Model file for the job. Use its own axes, mm. Give positions to 0.01 mm unless a question says otherwise; leave off trailing zeros. Write each loop counter-clockwise with the first axis right and the second up, starting at its lowest first coordinate (ties: lowest second). Pieces come first, ordered by that corner, then holes. Notation, with made-up numbers: (87, 55) - (100, 55) arc R21 cw to (100, 66) - close; hole circle Ø6 at (41.5, 53). An arc over 180 degrees is marked (long way). Use a Markdown table: item, result. Add a question column.
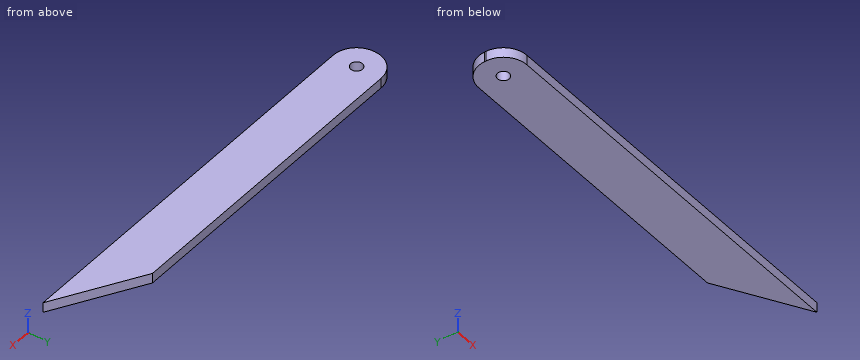
```python
from build123d import *

# Parameters (mm, degrees)
F1_DEPTH = 1.0795
F2_R     = 5.08
F3_R     = 1.27
F4_DEPTH = 25.4


with BuildPart() as f1:
    # F0 (on Top) → F1 (new body, symmetric)
    with BuildSketch(Plane.XY):
        Polygon((0, 10.414), (0, 0), (88.9, 0), (71.12, 10.414), align=None)
    extrude(amount=F1_DEPTH, both=True)

    # F2
    f2_edges = [f1.edges().sort_by_distance(p)[0] for p in [
        (0, 10.414, 0),
        (0, 0, 0),
    ]]
    fillet(f2_edges, radius=F2_R)

    # F3 (on face) → F4 (cut)
    with BuildSketch(Plane.XY.offset(1.0795)):
        with Locations((5.08, 5.08)):
            Circle(F3_R)
    extrude(amount=-F4_DEPTH, mode=Mode.SUBTRACT)


solid = f1.part
```
(1) Band-saw the part on B-B (y = 9). Write the cut outline in (x, z), then the cut area to 3 significant figures.
(2) Probe probe 1 along Y at (x, z) = (5.08, 0.45); probe 2 along X at (y, z) = (4.5, 0.2); probe 3 along X at (y, z) = (4.25, 0.9). List the from-to ranges inside material, lowest first. Write a range as [from, to].
(3) Flat gauge pin, fed straight in: pin 1 (1 mm diameter, centred on y = 2, z = -0.5, fed in from +X). Where does the tip first touch, or does it go through?
(4) Band-saw the part on A-A (z = 0.1). Write the cut outline in (x, y).
(5) Band-saw the part on C-C (x = 76.5). Write the cut outline in (y, z).
Model answer:
| question | item | result |
|---|---|---|
| 1 | outline | (1.56, -1.08) - (73.53, -1.08) - (73.53, 1.08) - (1.56, 1.08) - close |
| 1 | area | 155 mm^2 |
| 2 | probe 1 | y = [0, 3.81], [6.35, 10.41] |
| 2 | probe 2 | x = [0.03, 3.95], [6.21, 81.22] |
| 2 | probe 3 | x = [0.07, 4.12], [6.04, 81.64] |
| 3 | pin 1 | stops at x = 86.34 |
| 4 | outline | (0, 5.08) arc R5.08 ccw to (5.08, 0) - (88.9, 0) - (71.12, 10.41) - (5.08, 10.41) arc R5.08 ccw to (0, 5.33) - close; hole circle Ø2.54 at (5.08, 5.08) |
| 5 | outline | (0, -1.08) - (7.26, -1.08) - (7.26, 1.08) - (0, 1.08) - close |
